```python
from build123d import *

# Parameters (mm, degrees)
SKETCH_1_W               = 96
SKETCH_1_H               = 36
SKETCH_1_R               = 1.5
EXTRUDE_1_DEPTH          = 30
CUT_EXTRUDE_1_DEPTH      = 107.826962889
CUT_EXTRUDE_1_DEPTH_BACK = 107.826962889
SKETCH_2_R               = 10.917502173


with BuildPart() as part:
    # 草图1 → 凸台-拉伸1 (new body)
    with BuildSketch(Plane(origin=(0, 0, 0), x_dir=(1, 0, 0), z_dir=(0, 1, 0))):
        with Locations((48, 18)):
            Rectangle(SKETCH_1_W, SKETCH_1_H)
        with Locations(Location((10, 26, 0), (0, 0, 270))):
            Circle(SKETCH_1_R, mode=Mode.SUBTRACT)
        with Locations(Location((25, 26, 0), (0, 0, 270))):
            Circle(SKETCH_1_R, mode=Mode.SUBTRACT)
        with Locations(Location((25, 10, 0), (0, 0, 270))):
            Circle(SKETCH_1_R, mode=Mode.SUBTRACT)
        with Locations(Location((10, 10, 0), (0, 0, 270))):
            Circle(SKETCH_1_R, mode=Mode.SUBTRACT)
        with Locations(Location((86, 26, 0), (0, 0, 90))):
            Circle(SKETCH_1_R, mode=Mode.SUBTRACT)
        with Locations(Location((86, 10, 0), (0, 0, 90))):
            Circle(SKETCH_1_R, mode=Mode.SUBTRACT)
        with Locations(Location((71, 10, 0), (0, 0, 90))):
            Circle(SKETCH_1_R, mode=Mode.SUBTRACT)
        with Locations(Location((71, 26, 0), (0, 0, 90))):
            Circle(SKETCH_1_R, mode=Mode.SUBTRACT)
    extrude(amount=EXTRUDE_1_DEPTH)

    # 草图2 → 切除-拉伸1 (cut, two sides: drawn at the far end of the back side and taken through both)
    with BuildSketch(Plane(origin=(0, 0, -36), x_dir=(-1, 0, 0), z_dir=(0, 0, -1)).offset(-CUT_EXTRUDE_1_DEPTH_BACK)):
        with Locations((-48, 15)):
            Circle(SKETCH_2_R)
    extrude(amount=CUT_EXTRUDE_1_DEPTH + CUT_EXTRUDE_1_DEPTH_BACK, mode=Mode.SUBTRACT)


solid = part.part
```
Read the model definition and answer for the solid it produces. Units are mm, in the model's axes. Give positions to 0.01 mm unless a question says otherwise; leave off trailing zeros. Loops run counter-clockwise (first coordinate to the right, second up) from the corner with the lowest first, then second, coordinate; pieces in that order, holes last.
Item 1: Find the intervals of material crossed by line 1 along Z through (x, y) = (71, 11); line 2 along X through (y, z) = (25, -26); line 3 along X through (y, z) = (6.75, -26), in increasing order.
Item 2: The mould has two halves that part along Z. Classify faces 1 (the flat face through (47, 30, -18)), 2 (the flat face through (36.7, 14.8, -36)), 3 (the cylindrical face through (69.513, 14.79, -25.805)), 4 (the cylindrical face through (26.487, 14.79, -10.195)): released by +Z, released by -Z, zero draft, split by the parting line, or undercut.
Item 3: The part is cut by section A-A (z = -26). Write down the section's boundary in (x, y) (1 decimal), and give its area (3 significant figures).
Item 4: The part is cut by section C-C (x = 48). Write down the section's boundary in (y, z).
Item 5: The part is cut by section B-B (y = 15). Give the number of separate pieces and of enclosed holes in the cut face, and give its area (3 significant figures).
Taken from the geometry:
1. line 1: z = -36 to -27.5, -24.5 to -11.5, -8.5 to 0
1. line 2: x = 0 to 8.5, 11.5 to 23.5, 26.5 to 43.62, 52.38 to 69.5, 72.5 to 84.5, 87.5 to 96
1. line 3: x = 0 to 8.5, 11.5 to 23.5, 26.5 to 40.85, 55.15 to 69.5, 72.5 to 84.5, 87.5 to 96
2. face 1: zero draft
2. face 2: released by -Z
2. face 3: undercut
2. face 4: undercut
3. outline: (0, 0) - (8.5, 0) - (8.5, 30) - (0, 30) - close; (11.5, 0) - (23.5, 0) - (23.5, 30) - (11.5, 30) - close; (26.5, 0) - (69.5, 0) - (69.5, 30) - (26.5, 30) - close; (72.5, 0) - (84.5, 0) - (84.5, 30) - (72.5, 30) - close; (87.5, 0) - (96, 0) - (96, 30) - (87.5, 30) - close; hole circle Ø21.8 at (48, 15)
3. area: 2,150 mm2
4. outline: (0, -36) - (4.08, -36) - (4.08, 0) - (0, 0) - close; (25.92, -36) - (30, -36) - (30, 0) - (25.92, 0) - close
5. separate pieces: 2
5. enclosed holes: 8
5. area: 2,610 mm2
